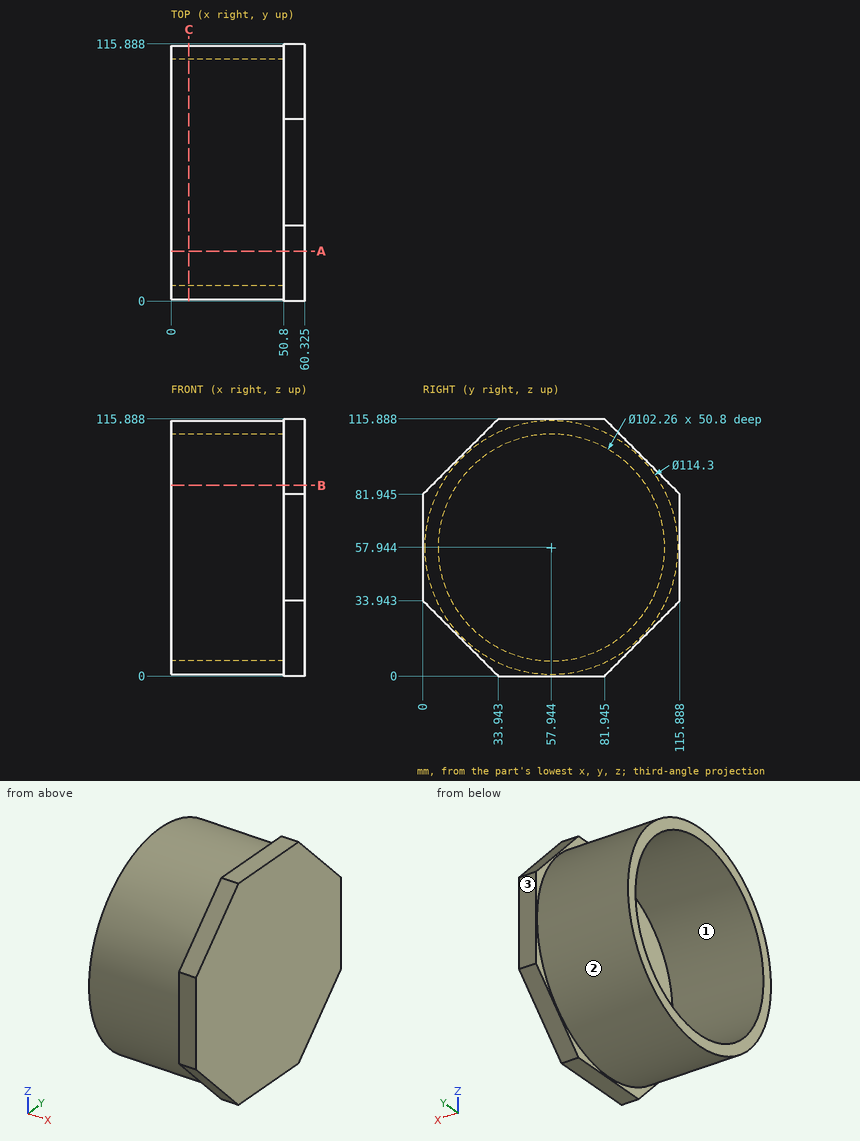
The drawing under review shows one solid part. Ordinate dimensions are in mm from its lowest x, y, z. Coordinates: 2 decimals unless noted, no trailing zeros. Order: outer loops, then holes, each group sorted by start corner. A loop starts at its lowest first (then second) coordinate and runs counter-clockwise, first axis right, second up. Notation, with made-up numbers: (11.5, 0) -> (45.5, 0) arc R22 cw to (45.5, 18) -> close; hole circle Ø8 at (82.25, -13). An arc over 180 degrees is marked (long way). Answer in a Markdown table with one row per item. Add a question column.
Item 1: To check wall thickness, follow probe 1 along X at (y, z) = (68, 63) (1 decimal); probe 2 along Z at (x, y) = (42.5, 88.5); probe 3 along Z at (x, y) = (48, 52.5) (1 decimal). State the ranges of each line that lie inside material, in increasing order.
Item 2: We need section C-C on x = 8. Write out the cut boundary in (y, z), plus the area to 3 significant figures.
Item 3: Clearance check with flat-ended pins moving along their axes: pin 1 (4 mm diameter, centred on x = 13, z = 77.5, fed in from -Y); pin 2 (1 mm diameter, centred on x = 8, z = 57, fed in from +Y); pin 3 (3 mm diameter, centred on x = 49, y = 69.5, fed in from +Z). State where each tip first meets the part, or that it passes through.
Item 4: We need section A-A on y = 22.5. Write out the cut boundary in (x, z) (1 decimal), plus the area to 3 significant figures.
Item 5: Mouldability with a two-part tool opening along Z and no side actions: class the marked faces 1, 2 and 3 as +Z half, -Z half, draft (parallel to the pull), parting line (faces both ways), or undercut.
Item 6: We need section B-B on z = 86. Write out the cut boundary in (x, y) (1 decimal), plus the area to 3 significant figures.
Final values:
| question | item | result |
|---|---|---|
| 1 | probe 1 | x = 50.8 to 60.3 |
| 1 | probe 2 | z = 9.65 to 16.95, 98.94 to 106.24 |
| 1 | probe 3 | z = 1.1 to 7.1, 108.8 to 114.8 |
| 2 | outline | circle Ø114.3 at (57.94, 57.94); hole circle Ø102.26 at (57.94, 57.94) |
| 2 | area | 2,050 mm2 |
| 3 | pin 1 | stops at y = 3.56 |
| 3 | pin 2 | stops at y = 115.09 |
| 3 | pin 3 | stops at z = 114.2 |
| 4 | outline | (0, 13.1) -> (50.8, 13.1) -> (50.8, 11.4) -> (60.3, 11.4) -> (60.3, 104.4) -> (50.8, 104.4) -> (50.8, 102.8) -> (0, 102.8) -> (0, 94.8) -> (50.8, 94.8) -> (50.8, 21.1) -> (0, 21.1) -> close |
| 4 | area | 1,700 mm2 |
| 5 | face 1 | undercut |
| 5 | face 2 | parting line |
| 5 | face 3 | draft |
| 6 | outline | (0, 8.2) -> (50.8, 8.2) -> (50.8, 4.1) -> (60.3, 4.1) -> (60.3, 111.8) -> (50.8, 111.8) -> (50.8, 107.7) -> (0, 107.7) -> (0, 100.7) -> (50.8, 100.7) -> (50.8, 15.2) -> (0, 15.2) -> close |
| 6 | area | 1,740 mm2 |
